```python
from build123d import *

# Parameters (mm, degrees)
SKETCH1_W           = 140
SKETCH1_H           = 70
BOSS_EXTRUDE1_DEPTH = 3.175
CUT_EXTRUDE1_DEPTH  = 4.175
CUT_EXTRUDE2_DEPTH  = 4.175


with BuildPart() as part:
    # Sketch1 → Boss-Extrude1 (new body)
    with BuildSketch(Plane.XY):
        with Locations((70, 35)):
            Rectangle(SKETCH1_W, SKETCH1_H)
    extrude(amount=BOSS_EXTRUDE1_DEPTH)

    # Sketch4 → Cut-Extrude1 (cut, through all)
    with BuildSketch(Plane.XY.offset(3.175)):
        Polygon((12.579717356, 63.555712168), (11.824972296, 60.471723696), (21.538321814, 58.094573903), (22.293066874, 61.178562375), align=None)
        Polygon((41.71976591, 56.424262788), (32.006416392, 58.801412581), (31.251671332, 55.71742411), (40.96502085, 53.340274316), align=None)
        Polygon((61.146464946, 51.669963201), (51.433115428, 54.047112995), (50.678370368, 50.963124523), (60.391719886, 48.585974729), align=None)
        Polygon((118.461678186, 11.905426097), (128.175027704, 9.528276304), (127.420282644, 6.444287832), (117.706933126, 8.821437625), align=None)
        Polygon((98.28023409, 13.575737212), (99.03497915, 16.659725684), (108.748328668, 14.28257589), (107.993583608, 11.198587419), align=None)
        Polygon((78.853535054, 18.330036799), (79.608280114, 21.414025271), (89.321629632, 19.036875477), (88.566884572, 15.952887005), align=None)
    extrude(amount=-CUT_EXTRUDE1_DEPTH, mode=Mode.SUBTRACT)

    # Sketch5 → Cut-Extrude2 (cut, through all)
    with BuildSketch(Plane.XY.offset(3.175)):
        Polygon((4.809647436, 70), (74.397727118, 52.969696608), (74.397727118, 27.23192206), (140, 11.177065891), (140, 70), align=None)
    extrude(amount=-CUT_EXTRUDE2_DEPTH, mode=Mode.SUBTRACT)


solid = part.part
```
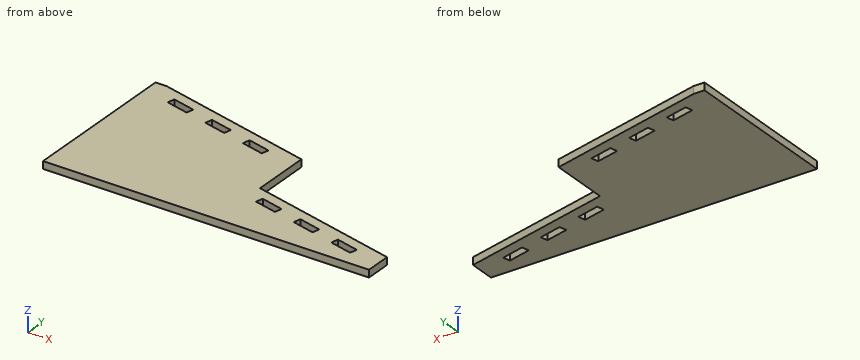
Geometry check sheet. Reference: the model listing, model coordinates, mm. Round coordinates to 2 decimals unless told otherwise and drop trailing zeros. Loops run counter-clockwise (first coordinate to the right, second up) from the corner with the lowest first, then second, coordinate; pieces in that order, holes last. Notation, with made-up numbers: (46.25, 45) - (73.25, 45) arc R28 cw to (73.25, 71) - close; hole circle Ø3 at (-9, 28.25). An arc over 180 degrees is marked (long way). Write item = value, one per line. Start each with the question number.
1. Thickness scan on line 1 (Y direction, x = 74.5, z = 0.3); line 2 (Y direction, x = 18.5, z = 1.1); line 3 (Y direction, x = 125.5, z = 0.9). Record the ranges inside material, lowest first.
2. Section check D-D on y = 32. Enter the section's corners in (x, z) (3 decimals).
3. Depth check by flat-ended pin: pin 1 (1.6 mm diameter, centred on y = 43.5, z = 1, fed in from +X); pin 2 (1 mm diameter, centred on x = 93.5, z = 2, fed in from +Y). Enter the tip coordinate at first touch or a pass-through.
4. Section check A-A on x = 35.5. Enter the section's corners in (y, z) (3 decimals).
5. Section check B-B on z = 1.4. Give the number of separate pieces and of enclosed holes in the cut face, then the cut area to 3 significant figures.
6. Section check C-C on x = 83.5. Enter the section's corners in (y, z) (3 decimals), then the cut area to 3 significant figures.
Working result:
q1.line_1 = 0 to 27.21
q1.line_2 = 0 to 58.84, 62.11 to 66.65
q1.line_3 = 0 to 6.91, 10.18 to 14.73
q2.outline = (0, 0) - (74.398, 0) - (74.398, 3.175) - (0, 3.175) - close
q3.pin_1 = 74.4
q3.pin_2 = 22.68
q4.outline = (0, 0) - (54.678, 0) - (54.678, 3.175) - (0, 3.175) - close; (57.946, 0) - (62.489, 0) - (62.489, 3.175) - (57.946, 3.175) - close
q5.separate_pieces = 1
q5.enclosed_holes = 6
q5.area = 5,680 mm^2
q6.outline = (0, 0) - (17.193, 0) - (17.193, 3.175) - (0, 3.175) - close; (20.462, 0) - (25.004, 0) - (25.004, 3.175) - (20.462, 3.175) - close
q6.area = 69.0 mm^2
